Design review of the part built by this model. Coordinates are the model's own, in mm. Coordinates: 2 decimals unless noted, no trailing zeros. Order: outer loops, then holes, each group sorted by start corner. A loop starts at its lowest first (then second) coordinate and runs counter-clockwise, first axis right, second up. Notation, with made-up numbers: (82.25, -13) - (128.25, -13) arc R17 cw to (128.25, 1) - close; hole circle Ø9 at (36, 56.25). An arc over 180 degrees is marked (long way). Write each question's results on one line, items separated by ' | '. Start each with the question number.
```python
from build123d import *

# Parameters (mm, degrees)
BOSS_EXTRU_1_DEPTH           = 8
ESQUISSE3_W                  = 20.3
ESQUISSE3_H                  = 8
ENL_V_MAT_EXTRU_1_DEPTH      = 8
ENL_V_MAT_EXTRU_2_DEPTH      = 10
ENL_V_MAT_EXTRU_3_DEPTH      = 757.11943364
ENL_V_MAT_EXTRU_3_DEPTH_BACK = 10
ESQUISSE5_W                  = 8
ESQUISSE5_H                  = 150
ESQUISSE5_H_2                = 12
ESQUISSE5_H_3                = 90
ESQUISSE5_H_4                = 30.343253
BOSS_EXTRU_2_DEPTH           = 8
ESQUISSE7_R                  = 19.05
ENL_V_MAT_EXTRU_4_DEPTH      = 10
ESQUISSE8_R                  = 2.8
ENL_V_MAT_EXTRU_5_DEPTH      = 10
ESQUISSE9_R                  = 3.15
ENL_V_MAT_EXTRU_6_DEPTH      = 10
ESQUISSE10_R                 = 2.65
ENL_V_MAT_EXTRU_7_DEPTH      = 10
ESQUISSE12_W                 = 60
ESQUISSE12_H                 = 8
ENL_V_MAT_EXTRU_8_DEPTH      = 10
ESQUISSE13_R                 = 2.6
ENL_V_MAT_EXTRU_9_DEPTH      = 10
ESQUISSE15_R                 = 2.6
ENL_V_MAT_EXTRU_10_DEPTH     = 10
ESQUISSE16_R                 = 2.6
ENL_V_MAT_EXTRU_11_DEPTH     = 10
ESQUISSE17_R                 = 4
ENL_V_MAT_EXTRU_12_DEPTH     = 10
ESQUISSE18_R                 = 2.1
ENL_V_MAT_EXTRU_13_DEPTH     = 10
ENL_V_MAT_EXTRU_14_DEPTH     = 10
ESQUISSE20_R                 = 25
ENL_V_MAT_EXTRU_15_DEPTH     = 10
BOSS_EXTRU_3_START           = -8
BOSS_EXTRU_3_DEPTH           = 8
ESQUISSE22_R                 = 7.5
ENL_V_MAT_EXTRU_16_DEPTH     = 10
ESQUISSE23_R                 = 2.6
ENL_V_MAT_EXTRU_17_DEPTH     = 10


with BuildPart() as part:
    # Esquisse2 → Boss.-Extru.1 (new body)
    with BuildSketch(Plane.XY.offset(-12)):
        Polygon((0, -56), (458.3, -56), (458.3, 601.343253), (0, 601.343253), (0, 571), (-8, 571), (-8, 556), (0, 556), (0, 466), (-8, 466), (-8, 451), (0, 451), (0, 301), (-8, 301), (-8, 286), (0, 286), (0, 136), (-8, 136), (-8, 121), (0, 121), (0, -29), (-8, -29), (-8, -44), (0, -44), align=None)
        with BuildLine():
            ThreePointArc((17, 53.829709717), (19.615223689, 56.884776311), (22.670290283, 59.5))
            Line((22.670290283, 59.5), (53.329709717, 59.5))
            ThreePointArc((53.329709717, 59.5), (56.384776311, 56.884776311), (59, 53.829709717))
            Line((59, 53.829709717), (59, 23.170290283))
            ThreePointArc((59, 23.170290283), (56.384776311, 20.115223689), (53.329709717, 17.5))
            Line((53.329709717, 17.5), (22.670290283, 17.5))
            ThreePointArc((22.670290283, 17.5), (19.615223689, 20.115223689), (17, 23.170290283))
            Line((17, 23.170290283), (17, 53.829709717))
        make_face(mode=Mode.SUBTRACT)
    extrude(amount=BOSS_EXTRU_1_DEPTH)

    # Esquisse3 → Enlèv. mat.-Extru.1 (cut)
    with BuildSketch(Plane.XY.offset(-4)):
        with Locations((163.483333333, 532)):
            Rectangle(ESQUISSE3_W, ESQUISSE3_H)
        with Locations((60.15, 532)):
            Rectangle(ESQUISSE3_W, ESQUISSE3_H)
        with Locations((266.816666667, 532)):
            Rectangle(ESQUISSE3_W, ESQUISSE3_H)
        with Locations((370.15, 532)):
            Rectangle(ESQUISSE3_W, ESQUISSE3_H)
    extrude(amount=-ENL_V_MAT_EXTRU_1_DEPTH, mode=Mode.SUBTRACT)

    # Esquisse4 → Enlèv. mat.-Extru.2 (cut)
    with BuildSketch(Plane.XY.offset(-4)):
        Polygon((358.3, 601.343253), (340.979491924, 591.343253), (117.320508076, 591.343253), (100, 601.343253), align=None)
    extrude(amount=-ENL_V_MAT_EXTRU_2_DEPTH, mode=Mode.SUBTRACT)

    # Esquisse5 → Enlèv. mat.-Extru.3 (cut, two sides: drawn at the far end of the back side and taken through both)
    with BuildSketch(Plane.XY.offset(-4).offset(-ENL_V_MAT_EXTRU_3_DEPTH_BACK)):
        with Locations((454.3, 46)):
            Rectangle(ESQUISSE5_W, ESQUISSE5_H)
        with Locations((454.3, -50)):
            Rectangle(ESQUISSE5_W, ESQUISSE5_H_2)
        with Locations((454.3, 211)):
            Rectangle(ESQUISSE5_W, ESQUISSE5_H)
        with Locations((454.3, 376)):
            Rectangle(ESQUISSE5_W, ESQUISSE5_H)
        with Locations((454.3, 511)):
            Rectangle(ESQUISSE5_W, ESQUISSE5_H_3)
        with Locations((454.3, 586.1716265)):
            Rectangle(ESQUISSE5_W, ESQUISSE5_H_4)
    extrude(amount=ENL_V_MAT_EXTRU_3_DEPTH + ENL_V_MAT_EXTRU_3_DEPTH_BACK, mode=Mode.SUBTRACT)

    # Esquisse6 → Boss.-Extru.2 (add)
    with BuildSketch(Plane.XY.offset(-12)):
        with BuildLine():
            Line((17, 53.829709717), (17, 23.170290283))
            ThreePointArc((17, 23.170290283), (19.615223689, 20.115223689), (22.670290283, 17.5))
            Line((22.670290283, 17.5), (53.329709717, 17.5))
            ThreePointArc((53.329709717, 17.5), (56.384776311, 20.115223689), (59, 23.170290283))
            Line((59, 23.170290283), (59, 53.829709717))
            ThreePointArc((59, 53.829709717), (56.384776311, 56.884776311), (53.329709717, 59.5))
            Line((53.329709717, 59.5), (22.670290283, 59.5))
            ThreePointArc((22.670290283, 59.5), (19.615223689, 56.884776311), (17, 53.829709717))
        make_face()
        with BuildLine():
            ThreePointArc((55, 38.5), (38, 55.5), (21, 38.5))
            ThreePointArc((21, 38.5), (38, 21.5), (55, 38.5))
        make_face(mode=Mode.SUBTRACT)
        with BuildLine():
            ThreePointArc((25.400757595, 53.349242405), (23.150757595, 55.599242405), (20.900757595, 53.349242405))
            ThreePointArc((20.900757595, 53.349242405), (23.150757595, 51.099242405), (25.400757595, 53.349242405))
        make_face(mode=Mode.SUBTRACT)
        with BuildLine():
            ThreePointArc((50.599242405, 53.349242405), (52.849242405, 51.099242405), (55.099242405, 53.349242405))
            ThreePointArc((55.099242405, 53.349242405), (52.849242405, 55.599242405), (50.599242405, 53.349242405))
        make_face(mode=Mode.SUBTRACT)
        with BuildLine():
            ThreePointArc((55.099242405, 23.650757595), (52.849242405, 25.900757595), (50.599242405, 23.650757595))
            ThreePointArc((50.599242405, 23.650757595), (52.849242405, 21.400757595), (55.099242405, 23.650757595))
        make_face(mode=Mode.SUBTRACT)
        with BuildLine():
            ThreePointArc((25.400757595, 23.650757595), (23.150757595, 25.900757595), (20.900757595, 23.650757595))
            ThreePointArc((20.900757595, 23.650757595), (23.150757595, 21.400757595), (25.400757595, 23.650757595))
        make_face(mode=Mode.SUBTRACT)
    extrude(amount=BOSS_EXTRU_2_DEPTH)

    # Esquisse7 → Enlèv. mat.-Extru.4 (cut)
    with BuildSketch(Plane.XY.offset(-4)):
        with Locations((38, 119.5)):
            Circle(ESQUISSE7_R)
    extrude(amount=-ENL_V_MAT_EXTRU_4_DEPTH, mode=Mode.SUBTRACT)

    # Esquisse8 → Enlèv. mat.-Extru.5 (cut)
    with BuildSketch(Plane.XY.offset(-4)):
        with Locations((61.55, 143.05)):
            Circle(ESQUISSE8_R)
        with Locations((14.45, 143.05)):
            Circle(ESQUISSE8_R)
        with Locations((14.45, 95.95)):
            Circle(ESQUISSE8_R)
        with Locations((61.55, 95.95)):
            Circle(ESQUISSE8_R)
    extrude(amount=-ENL_V_MAT_EXTRU_5_DEPTH, mode=Mode.SUBTRACT)

    # Esquisse9 → Enlèv. mat.-Extru.6 (cut)
    with BuildSketch(Plane.XY.offset(-4)):
        with Locations((426.5, 48.5)):
            Circle(ESQUISSE9_R)
        with Locations((426.5, 8.5)):
            Circle(ESQUISSE9_R)
    extrude(amount=-ENL_V_MAT_EXTRU_6_DEPTH, mode=Mode.SUBTRACT)

    # Esquisse10 → Enlèv. mat.-Extru.7 (cut)
    with BuildSketch(Plane.XY.offset(-4)):
        with Locations((251.15, 69.5)):
            Circle(ESQUISSE10_R)
        with Locations((199.15, 69.5)):
            Circle(ESQUISSE10_R)
    extrude(amount=-ENL_V_MAT_EXTRU_7_DEPTH, mode=Mode.SUBTRACT)

    # Esquisse12 → Enlèv. mat.-Extru.8 (cut)
    with BuildSketch(Plane(origin=(0, 0, -12), x_dir=(-1, 0, 0), z_dir=(0, 0, -1))):
        with Locations((-375.3, -52)):
            Rectangle(ESQUISSE12_W, ESQUISSE12_H)
        with Locations((-225.3, -52)):
            Rectangle(ESQUISSE12_W, ESQUISSE12_H)
        with Locations((-75.3, -52)):
            Rectangle(ESQUISSE12_W, ESQUISSE12_H)
    extrude(amount=-ENL_V_MAT_EXTRU_8_DEPTH, mode=Mode.SUBTRACT)

    # Esquisse13 → Enlèv. mat.-Extru.9 (cut)
    with BuildSketch(Plane.XY.offset(-4)):
        with Locations((312.3, -38)):
            Circle(ESQUISSE13_R)
        with Locations((290.3, -38)):
            Circle(ESQUISSE13_R)
        with Locations((164.3, -38)):
            Circle(ESQUISSE13_R)
        with Locations((142.3, -38)):
            Circle(ESQUISSE13_R)
    extrude(amount=-ENL_V_MAT_EXTRU_9_DEPTH, mode=Mode.SUBTRACT)

    # Esquisse15 → Enlèv. mat.-Extru.10 (cut)
    with BuildSketch(Plane(origin=(0, 0, -12), x_dir=(-1, 0, 0), z_dir=(0, 0, -1))):
        with Locations((-435.3, 378)):
            Circle(ESQUISSE15_R)
        with Locations((-435.3, 400)):
            Circle(ESQUISSE15_R)
        with Locations((-15, 378)):
            Circle(ESQUISSE15_R)
        with Locations((-15, 400)):
            Circle(ESQUISSE15_R)
    extrude(amount=-ENL_V_MAT_EXTRU_10_DEPTH, mode=Mode.SUBTRACT)

    # Esquisse16 → Enlèv. mat.-Extru.11 (cut)
    with BuildSketch(Plane.XY.offset(-4)):
        with Locations((337.15, 146)):
            Circle(ESQUISSE16_R)
        with Locations((113.15, 146)):
            Circle(ESQUISSE16_R)
        with Locations((113.15, -8)):
            Circle(ESQUISSE16_R)
        with Locations((337.15, -8)):
            Circle(ESQUISSE16_R)
    extrude(amount=-ENL_V_MAT_EXTRU_11_DEPTH, mode=Mode.SUBTRACT)

    # Esquisse17 → Enlèv. mat.-Extru.12 (cut)
    with BuildSketch(Plane.XY.offset(-4)):
        with Locations((20, 586.343253)):
            Circle(ESQUISSE17_R)
        with Locations((50, 586.343253)):
            Circle(ESQUISSE17_R)
        with Locations((400.3, 586.343253)):
            Circle(ESQUISSE17_R)
        with Locations((430.3, 586.343253)):
            Circle(ESQUISSE17_R)
    extrude(amount=-ENL_V_MAT_EXTRU_12_DEPTH, mode=Mode.SUBTRACT)

    # Esquisse18 → Enlèv. mat.-Extru.13 (cut)
    with BuildSketch(Plane(origin=(0, 0, -12), x_dir=(-1, 0, 0), z_dir=(0, 0, -1))):
        with Locations((-167, 90)):
            Circle(ESQUISSE18_R)
        with Locations((-167, 83)):
            Circle(ESQUISSE18_R)
        with Locations((-283.3, 470.5)):
            Circle(ESQUISSE18_R)
        with Locations((-283.3, 463.5)):
            Circle(ESQUISSE18_R)
    extrude(amount=-ENL_V_MAT_EXTRU_13_DEPTH, mode=Mode.SUBTRACT)

    # Esquisse19 → Enlèv. mat.-Extru.14 (cut)
    with BuildSketch(Plane.XY.offset(-4)):
        with BuildLine():
            Line((11.65, 143.05), (11.65, 150.05))
            ThreePointArc((11.65, 150.05), (14.45, 152.85), (17.25, 150.05))
            Line((17.25, 150.05), (17.25, 143.05))
            ThreePointArc((17.25, 143.05), (14.45, 140.25), (11.65, 143.05))
        make_face()
        with BuildLine():
            Line((58.75, 143.05), (58.75, 150.05))
            ThreePointArc((58.75, 150.05), (61.55, 152.85), (64.35, 150.05))
            Line((64.35, 150.05), (64.35, 143.05))
            ThreePointArc((64.35, 143.05), (61.55, 140.25), (58.75, 143.05))
        make_face()
        with BuildLine():
            Line((58.75, 95.95), (58.75, 102.95))
            ThreePointArc((58.75, 102.95), (61.55, 105.75), (64.35, 102.95))
            Line((64.35, 102.95), (64.35, 95.95))
            ThreePointArc((64.35, 95.95), (61.55, 93.15), (58.75, 95.95))
        make_face()
        with BuildLine():
            Line((11.65, 95.95), (11.65, 102.95))
            ThreePointArc((11.65, 102.95), (14.45, 105.75), (17.25, 102.95))
            Line((17.25, 102.95), (17.25, 95.95))
            ThreePointArc((17.25, 95.95), (14.45, 93.15), (11.65, 95.95))
        make_face()
    extrude(amount=-ENL_V_MAT_EXTRU_14_DEPTH, mode=Mode.SUBTRACT)

    # Esquisse20 → Enlèv. mat.-Extru.15 (cut)
    with BuildSketch(Plane.XY.offset(-4)):
        with Locations((108, 360.5)):
            Circle(ESQUISSE20_R)
    extrude(amount=-ENL_V_MAT_EXTRU_15_DEPTH, mode=Mode.SUBTRACT)

    # Esquisse21 → Boss.-Extru.3 (add)
    with BuildSketch(Plane(origin=(0, 0, -12), x_dir=(-1, 0, 0), z_dir=(0, 0, -1)).offset(BOSS_EXTRU_3_START)):
        with BuildLine():
            Line((-90.650648427, 378.5), (-125.349351573, 378.5))
            ThreePointArc((-125.349351573, 378.5), (-108, 385.5), (-90.650648427, 378.5))
        make_face()
    extrude(amount=BOSS_EXTRU_3_DEPTH)

    # Esquisse22 → Enlèv. mat.-Extru.16 (cut)
    with BuildSketch(Plane(origin=(0, 0, -12), x_dir=(-1, 0, 0), z_dir=(0, 0, -1))):
        with Locations((-210, 471.343253)):
            Circle(ESQUISSE22_R)
        with Locations((-130, 72)):
            Circle(ESQUISSE22_R)
    extrude(amount=-ENL_V_MAT_EXTRU_16_DEPTH, mode=Mode.SUBTRACT)

    # Esquisse23 → Enlèv. mat.-Extru.17 (cut)
    with BuildSketch(Plane(origin=(0, 0, -12), x_dir=(-1, 0, 0), z_dir=(0, 0, -1))):
        with Locations((-435.3, 232)):
            Circle(ESQUISSE23_R)
        with Locations((-435.3, 210)):
            Circle(ESQUISSE23_R)
        with Locations((-15, 232)):
            Circle(ESQUISSE23_R)
        with Locations((-15, 210)):
            Circle(ESQUISSE23_R)
    extrude(amount=-ENL_V_MAT_EXTRU_17_DEPTH, mode=Mode.SUBTRACT)


solid = part.part
```
(1) To check wall thickness, follow line 1 along X through (y, z) = (528.5, -11.5); line 2 along Y through (x, z) = (435.3, -8.5); line 3 along Y through (x, z) = (312.3, -8.5). State the ranges of each line that lie inside material, in increasing order. Write a range as [from, to].
(2) Mouldability with a two-part tool opening along X and no side actions: class faces 1 (the face through (206.54, 464.69, -8.06)), 2 (the face through (222, 277, -4)) as +X half, -X half, draft (parallel to the pull), parting line (faces both ways), or undercut.
(3) Take a section at B-B (z = -6). State how many separate pieces and enclosed holes the cut face has, plus the area to 3 significant figures.
(4) Clearance check with flat-ended pins moving along their axes: pin 1 (2.5 mm diameter, centred on y = 530.5, z = -8.5, fed in from -X); pin 2 (4 mm diameter, centred on x = 454.5, z = -7, fed in from -Y); pin 3 (4 mm diameter, centred on x = 454, z = -7.5, fed in from +Y). State where each tip first meets the part, or that it passes through.
(5) Take a section at A-A (y = 416). State the section outline as (x, z) points.
Worked out:
1) line 1: [0, 50], [70.3, 153.33], [173.63, 256.67], [276.97, 360], [380.3, 450.3] | line 2: [-56, 207.4], [212.6, 229.4], [234.6, 375.4], [380.6, 397.4], [402.6, 601.34] | line 3: [-56, -40.6], [-35.4, 591.34]
2) face 1: undercut | face 2: draft
3) separate pieces: 1 | enclosed holes: 45 | area: 287,000 mm^2
4) pin 1: x = 0 | pin 2: y = -44 | pin 3: y = 571
5) outline: (0, -12) - (450.3, -12) - (450.3, -4) - (0, -4) - close
